Part model, mm, in its own coordinate system. A direction names the side the tool comes from. Give positions to 0.01 mm unless a question says otherwise; leave off trailing zeros. Loops run counter-clockwise (first coordinate to the right, second up) from the corner with the lowest first, then second, coordinate; pieces in that order, holes last. Notation, with made-up numbers: M 32.5,18.5 L 75.5,18.5 A11 cw 75.5,33.5 Z; hole C 16,73 d9. An arc over 180 degrees is marked long. Answer in a Markdown table with one row per item.
from build123d import *

# Parameters (mm, degrees)
BOSS_EXTRUDE1_DEPTH       = 22.5
F_3_0MM_DOWEL_HOLE1_D     = 3
BOSS_EXTRUDE2_START       = -8.493151603
BOSS_EXTRUDE2_OUTLINE_W   = 45
BOSS_EXTRUDE2_OUTLINE_H   = 45
BOSS_EXTRUDE2_DEPTH       = 40.493151603
SKETCH5_R                 = 17.5
CUT_EXTRUDE1_DEPTH        = 40.493152
SKETCH7_W                 = 10
SKETCH7_H                 = 45
CUT_EXTRUDE2_DEPTH        = 78.641837948
SKETCH8_W                 = 22.5
SKETCH8_H                 = 22.5
CUT_EXTRUDE3_DEPTH        = 10
CUT_EXTRUDE5_OUTLINE_W    = 1.5
CUT_EXTRUDE5_OUTLINE_H    = 5.064430618
CUT_EXTRUDE8_START        = 17.435595673
CUT_EXTRUDE8_DEPTH        = 5.064404327
SKETCH14_W                = 10
SKETCH14_H                = 15
BOSS_EXTRUDE3_DEPTH       = 5
M3X0_5_TAPPED_HOLE1_D     = 2.5
M3X0_5_TAPPED_HOLE1_DEPTH = 7.748924226
M3X0_5_TAPPED_HOLE1_TIP   = 0.751075774
CHAMFER1_SIZE             = 15
FILLET1_R                 = 2
FILLET2_R                 = 5
FILLET3_R                 = 5


# Read off the part's stored shape, not the designer's step: Boss-Extrude2, Cut-Extrude5, Cut-Extrude8
with BuildPart() as part:
    # Sketch3 → Boss-Extrude1 (new, symmetric)
    with BuildSketch(Plane(origin=(0, 0, 0), x_dir=(1, 0, 0), z_dir=(0, 1, 0))):
        with BuildLine():
            Line((-53.560989258, 0.75), (-53.560989258, 5.75))
            Line((-53.560989258, 5.75), (-33.560989258, 5.75))
            ThreePointArc((-33.560989258, 5.75), (34.05, 0), (-33.560989258, -5.75))
            Line((-33.560989258, -5.75), (-53.560989258, -5.75))
            Line((-53.560989258, -5.75), (-53.560989258, -0.75))
            Line((-53.560989258, -0.75), (-19.035230495, -0.75))
            ThreePointArc((-19.035230495, -0.75), (19.05, 0), (-19.035230495, 0.75))
            Line((-19.035230495, 0.75), (-53.560989258, 0.75))
        make_face()
    extrude(amount=BOSS_EXTRUDE1_DEPTH, both=True)

    # Ø3.0mm Dowel Hole1 (through all)
    with Locations(Plane.XY.offset(5.75)):
        with Locations((-43.560989258, 7.5), (-43.560989258, -7.5)):
            Hole(F_3_0MM_DOWEL_HOLE1_D / 2)

    # Boss-Extrude2 outline → Boss-Extrude2 (add)
    with BuildSketch(Plane(origin=(34.05, 0, 0), x_dir=(0, 0, -1), z_dir=(1, 0, 0)).offset(BOSS_EXTRUDE2_START)):
        Rectangle(BOSS_EXTRUDE2_OUTLINE_W, BOSS_EXTRUDE2_OUTLINE_H)
    extrude(amount=BOSS_EXTRUDE2_DEPTH)

    # Sketch5 → Cut-Extrude1 (cut)
    with BuildSketch(Plane(origin=(66.05, 0, 0), x_dir=(0, 0, -1), z_dir=(1, 0, 0))):
        Circle(SKETCH5_R)
    extrude(amount=-CUT_EXTRUDE1_DEPTH, mode=Mode.SUBTRACT)

    # Sketch7 → Cut-Extrude2 (cut, through all)
    with BuildSketch(Plane(origin=(0, 0, 0), x_dir=(1, 0, 0), z_dir=(0, 1, 0))):
        with Locations((41.05, 0)):
            Rectangle(SKETCH7_W, SKETCH7_H)
    extrude(amount=CUT_EXTRUDE2_DEPTH, mode=Mode.SUBTRACT)

    # Sketch8 → Cut-Extrude3 (cut)
    with BuildSketch(Plane(origin=(66.05, 0, 0), x_dir=(0, 0, -1), z_dir=(1, 0, 0))):
        with Locations((-11.25, 11.25)):
            Rectangle(SKETCH8_W, SKETCH8_H)
    extrude(amount=-CUT_EXTRUDE3_DEPTH, mode=Mode.SUBTRACT)

    # Cut-Extrude5 outline → Cut-Extrude5 (revolve, cut)
    with BuildSketch(Plane(origin=(57.55, 0, 0), x_dir=(1, 0, 0), z_dir=(0, -1, 0))):
        with Locations((0.75, 19.967784691)):
            Rectangle(CUT_EXTRUDE5_OUTLINE_W, CUT_EXTRUDE5_OUTLINE_H)
    revolve(axis=Axis((57.55, 0, 0), (0, 0, 1)), mode=Mode.SUBTRACT)

    # Cut-Extrude8 outline → Cut-Extrude8 (cut)
    with BuildSketch(Plane(origin=(0, 0, 0), x_dir=(1, 0, 0), z_dir=(0, 1, 0)).offset(CUT_EXTRUDE8_START)):
        with BuildLine():
            ThreePointArc((59.05, 0), (57.55, 1.5), (56.05, 0))
            Line((56.05, 0), (59.05, 0))
        make_face()
    extrude(amount=CUT_EXTRUDE8_DEPTH, mode=Mode.SUBTRACT)

    # Sketch14 → Boss-Extrude3 (add)
    with BuildSketch(Plane(origin=(0, 0, 0), x_dir=(1, 0, 0), z_dir=(0, 1, 0))):
        with Locations((41.05, -25)):
            Rectangle(SKETCH14_W, SKETCH14_H)
        with Locations((41.05, 25)):
            Rectangle(SKETCH14_W, SKETCH14_H)
    extrude(amount=-BOSS_EXTRUDE3_DEPTH)

    # M3x0.5 Tapped Hole1
    with Locations(Plane(origin=(0, 0, 0), x_dir=(1, 0, 0), z_dir=(0, 1, 0))):
        with Locations((41.05, 27.5), (41.05, -27.5)):
            Hole(M3X0_5_TAPPED_HOLE1_D / 2, depth=M3X0_5_TAPPED_HOLE1_DEPTH)
            with Locations((0, 0, -(M3X0_5_TAPPED_HOLE1_DEPTH + M3X0_5_TAPPED_HOLE1_TIP / 2))):  # 118° drill point
                Cone(0, M3X0_5_TAPPED_HOLE1_D / 2, M3X0_5_TAPPED_HOLE1_TIP, mode=Mode.SUBTRACT)

    # Chamfer1
    chamfer1_edges = [part.edges().sort_by_distance(p)[0] for p in [
        (51.05, 22.5, 22.5),
    ]]
    chamfer(chamfer1_edges, length=CHAMFER1_SIZE)

    # Fillet1
    fillet1_edges = [part.edges().sort_by_distance(p)[0] for p in [
        (41.05, -5, 22.5),
        (41.05, -5, -22.5),
    ]]
    fillet(fillet1_edges, radius=FILLET1_R)

    # Fillet2
    fillet2_edges = [part.edges().sort_by_distance(p)[0] for p in [
        (51.05, 22.5, 7.5),
        (51.05, 7.5, 22.5),
    ]]
    fillet(fillet2_edges, radius=FILLET2_R)

    # Fillet3
    fillet3_edges = [part.edges().sort_by_distance(p)[0] for p in [
        (-33.560989258, 0, -5.75),
        (-33.560989258, 0, 5.75),
        (25.556848397, 0, -22.5),
        (25.556848397, 0, 22.5),
    ]]
    fillet(fillet3_edges, radius=FILLET3_R)


solid = part.part
(1) Drill centre lines: line 1 along Z through (x, y) = (-47.5, -6); line 2 along Z through (x, y) = (41.05, -3.75); line 3 along X through (y, z) = (-3, 27). Where is each one in solid material? Low to high.
Recorded:
| item | result |
|---|---|
| line 1 | z = -5.75 to -0.75, 0.75 to 5.75 |
| line 2 | z = -32.5 to -28.75, -26.25 to -17.09, 17.09 to 26.25, 28.75 to 32.5 |
| line 3 | x = -20.75 to 20.75, 36.05 to 39.9, 42.2 to 46.05 |
(2) Pin check, flat tips, straight feed: pin 1 Ø4 at (x, z) = (41.5, 28.5) entering from -Y; pin 2 Ø3 at (x, y) = (-36.5, -15) entering from -Z; pin 3 Ø4 at (x, y) = (-43.56, 7.5) entering from -Z; pin 4 Ø3 at (x, z) = (17.5, 4) entering from +Y. Stop position of each tip, or through.
Recorded:
| item | result |
|---|---|
| pin 1 | stops at y = -5 |
| pin 2 | stops at z = -6.44 |
| pin 3 | stops at z = -5.75 |
| pin 4 | stops at y = 22.5 |
(3) Saw through at D-D (z = 27.5). Write the cut outline in (x, y), plus the area to 3 significant figures.
Recorded:
| item | result |
|---|---|
| outline | M -20.08,-22.5 L 20.08,-22.5 L 20.08,22.5 L -20.08,22.5 Z; M 36.05,-5 L 39.8,-5 L 39.8,0 L 36.05,0 Z; M 42.3,-5 L 46.05,-5 L 46.05,0 L 42.3,0 Z |
| area | 1,840 mm^2 |
(4) Pull direction Y, two halves, no side cores. Call faces 6 (the face through (41, -5, 29)), 7 (the face through (-43.236, 6.036, 3.215)), 8 (the face through (25.827, 0.315, 22.874)): +Y half, -Y half, draft (parallel to the pull), parting line (faces both ways), or undercut.
Recorded:
| item | result |
|---|---|
| face 6 | -Y half |
| face 7 | undercut |
| face 8 | draft |
(5) Saw through at A-A (x = 41.05). Write the cut outline in (y, z), plus the area to 3 significant figures.
Recorded:
| item | result |
|---|---|
| outline | M -22.5,-22.5 L -7,-22.5 A2 cw -5,-24.5 L -5,-26.25 L 0,-26.25 L 0,-17.5 A17.5 cw 0,17.5 L 0,26.25 L -5,26.25 L -5,24.5 A2 cw -7,22.5 L -22.5,22.5 Z; M -5,-32.5 L 0,-32.5 L 0,-28.75 L -5,-28.75 Z; M -5,28.75 L 0,28.75 L 0,32.5 L -5,32.5 Z |
| area | 608 mm^2 |
(6) Saw through at C-C (x = -6). Write the cut outline in (y, z).
Recorded:
| item | result |
|---|---|
| outline | M -22.5,-33.52 L 22.5,-33.52 L 22.5,-18.08 L -22.5,-18.08 Z; M -22.5,18.08 L 22.5,18.08 L 22.5,33.52 L -22.5,33.52 Z |
(7) Saw through at B-B (y = 10.5). Write the cut outline in (x, z), plus the area to 3 significant figures.
Recorded:
| item | result |
|---|---|
| outline | M -53.56,-5.75 L -37.54,-5.75 A5 cw -32.73,-9.37 A34.05 ccw 24.17,-23.98 A5 cw 27.72,-22.5 L 36.05,-22.5 L 36.05,-14 L 25.56,-14 L 25.56,14 L 36.05,14 L 36.05,22.5 L 27.72,22.5 A5 cw 24.17,23.98 A34.05 ccw -32.73,9.37 A5 cw -37.54,5.75 L -53.56,5.75 L -53.56,0.75 L -19.04,0.75 A19.05 cw long -19.04,-0.75 L -53.56,-0.75 Z; M 46.05,-22.5 L 66.05,-22.5 L 66.05,-14 L 46.05,-14 Z; M 46.05,14 L 56.05,14 L 56.05,19.5 L 46.05,19.5 Z |
| area | 2,830 mm^2 |
(8) Which spindle directions (+Z, -Z, +X, -X, +Y, -Y) get a long thin tool onto all of the face, cutting with end or side? Do faces 1 (the face through (46.087, -15.526, -8.075)), 2 (the face through (63, 20, 0)), 3 (the face through (46.05, 19, -5)), 4 (the face through (-46, 0, -5.75)), 5 (the face through (41, -2, -32.5)). Say none if no direction does.
Recorded:
| item | result |
|---|---|
| face 1 | +X |
| face 2 | +Z, +X, +Y |
| face 3 | +Z, -Z, +Y |
| face 4 | -Z, -X, +Y, -Y |
| face 5 | -Z, +X, +Y, -Y |
